The listing builds one solid part. Answer for the finished solid, in the listing's coordinates (mm). Face numbers are marked on the shaded views. A direction names the side the tool comes from. Round coordinates to 2 decimals unless told otherwise and drop trailing zeros. Loops run counter-clockwise (first coordinate to the right, second up) from the corner with the lowest first, then second, coordinate; pieces in that order, holes last. Notation, with made-up numbers: (-15.5, -15) - (6.5, -15) arc R20 ccw to (6.5, 19) - close; hole circle Ø4 at (85.5, 66). An arc over 180 degrees is marked (long way). One line per item, written item: value.
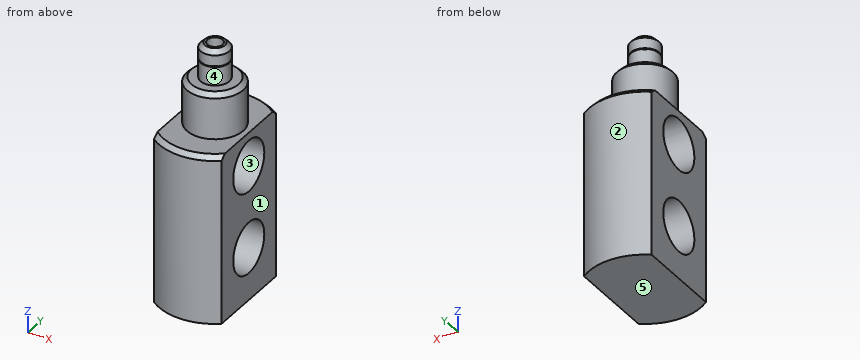
```python
from build123d import *

# Parameters (mm, degrees)
F0_R      = 25.4
F1_DEPTH  = 76.2
F2_R      = 12.7124561547
F3_DEPTH  = 20.574
F4_R      = 6.5036133295
F5_DEPTH  = 8.382
F6_R      = 5.5261881266
F7_DEPTH  = 0.3556
F8_R      = 6.0681325209
F9_DEPTH  = 0.5588
F10_R     = 6.5080423993
F11_DEPTH = 6.8072
F12_W     = 12.8267863765
F12_H     = 46.3458411396
F13_DEPTH = 254
F14_W     = 15.4017303139
F14_H     = 51.6813602298
F15_DEPTH = 254
F16_R     = 11.58530812
F17_DEPTH = 254
F18_R     = 11.5775255265
F19_DEPTH = 254
F20_SIZE  = 2.032
F21_SIZE  = 2.032
F24_R     = 3.4812427805
F25_DEPTH = 50.8


# Not quite as in the source:
# - two fillets or chamfers of one size are made in one step


with BuildPart() as f1:
    # F0 (on Top) → F1 (new body)
    with BuildSketch(Plane.XY):
        Circle(F0_R)
    extrude(amount=F1_DEPTH)

    # F2 (on face) → F3 (join)
    with BuildSketch(Plane.XY.offset(76.2)):
        Circle(F2_R)
    extrude(amount=F3_DEPTH)

    # F4 (on face) → F5 (join)
    with BuildSketch(Plane.XY.offset(96.774)):
        Circle(F4_R)
    extrude(amount=F5_DEPTH)

    # F6 (on face) → F7 (join)
    with BuildSketch(Plane.XY.offset(105.156)):
        Circle(F6_R)
    extrude(amount=-F7_DEPTH)

    # F8 (on face) → F9 (join)
    with BuildSketch(Plane.XY.offset(105.156)):
        Circle(F8_R)
    extrude(amount=F9_DEPTH)

    # F10 (on face) → F11 (join)
    with BuildSketch(Plane.XY.offset(105.7148)):
        Circle(F10_R)
    extrude(amount=F11_DEPTH)

    # F12 (on face) → F13 (cut)
    with BuildSketch(Plane.XY.offset(76.2)):
        with Locations((-21.7024399899, -0.1023318619)):
            Rectangle(F12_W, F12_H)
    extrude(amount=-F13_DEPTH, mode=Mode.SUBTRACT)

    # F14 (on face) → F15 (cut)
    with BuildSketch(Plane.XY.offset(76.2)):
        with Locations((22.9368926957, -0.5596792325)):
            Rectangle(F14_W, F14_H)
    extrude(amount=-F15_DEPTH, mode=Mode.SUBTRACT)

    # F16 (on face) → F17 (cut)
    with BuildSketch(Plane.YZ.offset(15.2360275388)):
        with Locations((0, 61.0498785973)):
            Circle(F16_R)
    extrude(amount=-F17_DEPTH, mode=Mode.SUBTRACT)

    # F18 (on face) → F19 (cut)
    with BuildSketch(Plane.YZ.offset(15.2360275388)):
        with Locations((0, 23.8405317068)):
            Circle(F18_R)
    extrude(amount=-F19_DEPTH, mode=Mode.SUBTRACT)

    # F20
    f20_edges = [f1.edges().sort_by_distance(p)[0] for p in [
        (-0.033165, 25.399978, 76.2),
        (-0.033165, -25.399978, 76.2),
    ]]
    chamfer(f20_edges, length=F20_SIZE)

    # F21
    f21_edges = [f1.edges().sort_by_distance(p)[0] for p in [
        (-12.712456, 0, 96.774),
        (-6.508042, 0, 112.522),
    ]]
    chamfer(f21_edges, length=F21_SIZE)

    # F24 (on face) → F25 (cut)
    with BuildSketch(Plane.XY.offset(112.522)):
        Circle(F24_R)
    extrude(amount=-F25_DEPTH, mode=Mode.SUBTRACT)


solid = f1.part
```
1) Consider L1, parallel to Z at x = 7.5, y = -10.5; L2, parallel to Z at x = 6, y = -5; L3, parallel to Z at x = 0, y = 1. Determine where each line is inside the solid, lowest interval first.
Final values:
L1: 0 to 18.96, 28.72 to 56.15, 65.95 to 76.2
L2: 0 to 13.4, 34.28 to 50.6, 71.5 to 96.77
L3: 0 to 12.31, 35.37 to 49.51
2) A cutting plane is placed at A-A on z = 26.5. Give the vertices of the cut face in (x, y), and give its area (3 significant figures).
Final values:
outline: (-15.29, -20.28) arc R25.4 ccw to (15.24, -20.32) - (15.24, -11.27) - (-15.29, -11.27) - close; (-15.29, 11.27) - (15.24, 11.27) - (15.24, 20.32) arc R25.4 ccw to (-15.29, 20.28) - close
area: 764 mm2
3) A cutting plane is placed at C-C on y = 0. Give the number of separate pieces and of enclosed holes in the cut face, and give its area (3 significant figures).
Final values:
separate pieces: 4
enclosed holes: 0
area: 1,350 mm2
4) For a pull along Y with two mould halves and no side action, classify the marked faces 1, 2 and 3 as released by +Y, released by -Y, zero draft, split by the parting line, or undercut.
Final values:
face 1: zero draft
face 2: released by +Y
face 3: undercut
5) For the marked faces 4 and 5, determine the directions among +Z, -Z, +X, -X, +Y, -Y from which every point of the face is accessible in a straight line to the end or side of a thin tool.
Final values:
face 4: +Z
face 5: -Z, +X, -X, +Y, -Y
6) Each of these flat-tipped pins is pushed along its axis until it touches: pin 1 Ø5 at (x, y) = (3, 12.5) entering from +Z; pin 2 Ø12 at (x, z) = (0, 59) entering from +Y; pin 3 Ø2 at (x, y) = (11, -12) entering from +Z; pin 4 Ø21 at (y, z) = (0, 61.05) entering from +X. Where does it stop, or does it pass through?
Final values:
pin 1: z = 96.77
pin 2: y = 25.4
pin 3: z = 76.2
pin 4: through
